Could you check a few things on this model? Use its own coordinates, in mm. Face numbers are marked on the shaded views. A direction names the side the tool comes from. Coordinates: 2 decimals unless noted, no trailing zeros. Loops run counter-clockwise (first coordinate to the right, second up) from the corner with the lowest first, then second, coordinate; pieces in that order, holes last. Notation, with made-up numbers: (47.5, 43) - (92.5, 43) arc R29 cw to (92.5, 69) - close; hole circle Ø3 at (60, -28). An arc over 180 degrees is marked (long way). One line per question, with ' | ' between items. Start each with the question number.
1. I want a section at A-A, the plane z = 13.5. Write out the boundary of the cut face in (x, y), then the cut area to 3 significant figures.
2. We'd pull the mould along X, two halves only. Please class the marked faces 1, 2 and 3: pulls with the +X half, pulls with the -X half, needs draft (parallel to the pull), parting line crosses it, or undercut.
3. I want a section at C-C, the plane x = 28. Write out the boundary of the cut face in (y, z), then the cut area to 3 significant figures.
4. Which directions (+Z, -Z, +X, -X, +Y, -Y) give clear straight access to the entire face, cutting with the end or side of a thin tool? Please do the marked faces 4 and 5.
5. I'm going to push a flat-ended pin straight in: P1, Ø17, axis at x = 44.5, y = 39.5, coming from the -Z side. Where does the tip first touch, or does it pass through?
6. I want a section at B-B, the plane y = 48.5. Write out the boundary of the cut face in (x, z).
7. Please list where these lines run through material, in increasing order: L1, parallel to X at y = 11.5, z = 22.5; L2, parallel to Y at x = 55.5, z = 21.5; L3, parallel to Z at x = 63.5, y = 24.5. Write a range as [from, to].
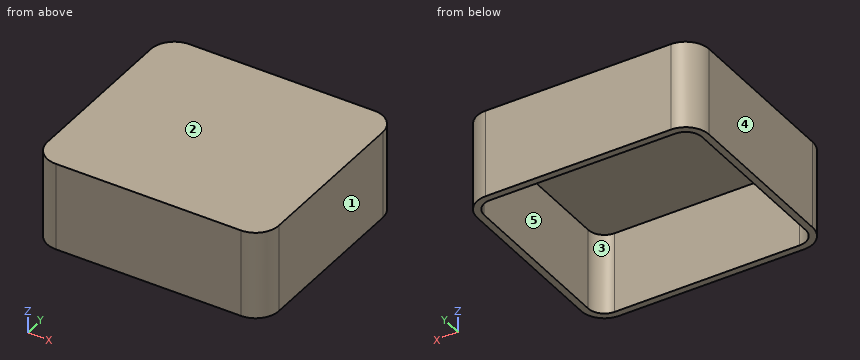
from build123d import *

# Parameters (mm, degrees)
EXTRUDE_DEPTH = 25
THICKNESS_T   = -2


with BuildPart() as part:
    # Sketch → Extrude (new body)
    with BuildSketch(Plane.XY):
        with BuildLine():
            Line((6.7, 0), (59.4, 0))
            ThreePointArc((59.4, 0), (64.066905, 1.933095), (66, 6.6))
            Line((66, 6.6), (66, 53.4))
            ThreePointArc((66, 53.4), (64.066905, 58.066905), (59.4, 60))
            Line((59.4, 60), (6.7, 60))
            ThreePointArc((6.7, 60), (1.962385, 58.037615), (0, 53.3))
            Line((0, 53.3), (0, 6.7))
            ThreePointArc((0, 6.7), (1.962385, 1.962385), (6.7, 0))
        make_face()
    extrude(amount=EXTRUDE_DEPTH)

    # Thickness
    thickness_openings = [part.faces().sort_by_distance(p)[0] for p in [
        (33.004479, 30, 0),
    ]]
    offset(amount=THICKNESS_T, openings=thickness_openings)


solid = part.part
Results are:
1) outline: (0, 6.7) arc R6.7 ccw to (6.7, 0) - (59.4, 0) arc R6.6 ccw to (66, 6.6) - (66, 53.4) arc R6.6 ccw to (59.4, 60) - (6.7, 60) arc R6.7 ccw to (0, 53.3) - close; hole (2, 6.7) arc R4.7 ccw to (6.7, 2) - (59.4, 2) arc R4.6 ccw to (64, 6.6) - (64, 53.4) arc R4.6 ccw to (59.4, 58) - (6.7, 58) arc R4.7 ccw to (2, 53.3) - close | area: 469 mm2
2) face 1: pulls with the +X half | face 2: needs draft | face 3: undercut
3) outline: (0, 0) - (2, 0) - (2, 23) - (58, 23) - (58, 0) - (60, 0) - (60, 25) - (0, 25) - close | area: 212 mm2
4) face 4: +Z, -Z, -X, +Y, -Y | face 5: -Z
5) P1: stops at z = 23
6) outline: (0, 0) - (2, 0) - (2, 23) - (64, 23) - (64, 0) - (66, 0) - (66, 25) - (0, 25) - close
7) L1: x = [0, 2], [64, 66] | L2: y = [0, 2], [58, 60] | L3: z = [23, 25]
